```python
from build123d import *

# Parameters (mm, degrees)
F2_R     = 10.5676667099
F3_DEPTH = 124.5231421123
F4_R     = 5.08


# Not quite as in the source:
# - a feature names something its author has since deleted; it is built from what else it names


with BuildPart() as f1:
    # F0 (on Front) → F1 (revolve)
    with BuildSketch(Plane.XZ):
        Polygon((0, 25.3843758255), (0, 0), (124.5221421123, 0), (124.5221421123, 11.6869108751), (108.956836164, 25.3843758255), (94.325453043, 25.3843758255), (94.325453043, 55.5810630322), (84.0523540974, 55.5810630322), (84.0523540974, 25.3843758255), (40.1582047343, 25.3843758255), (40.1582047343, 57.137593627), (28.951190412, 57.137593627), (28.951190412, 25.3843758255), align=None)
    revolve(axis=Axis((62.2610710561, 0, 0), (1, 0, 0)))

    # F2 (on Right) → F3 (cut, through all)
    with BuildSketch(Plane.YZ):
        Circle(F2_R)
    extrude(amount=F3_DEPTH, mode=Mode.SUBTRACT)

    # F4
    f4_edges = [f1.edges().sort_by_distance(p)[0] for p in [
        (108.956836, 0, -25.384376),
        (94.325453, 0, -55.581063),
        (28.95119, 0, -57.137594),
    ]]
    fillet(f4_edges, radius=F4_R)


solid = f1.part
```
Geometry: final body of the model. Coordinates: model frame, mm. A direction names the side the tool comes from. Give positions to 0.01 mm unless a question says otherwise; leave off trailing zeros. Write each loop counter-clockwise with the first axis right and the second up, starting at its lowest first coordinate (ties: lowest second). Pieces come first, ordered by that corner, then holes.
1. Reachability of faces 1 (the cylindrical face through (86.613, -16.695, 53.014)), 2 (the cylindrical face through (14.27, 24.78, -5.5)), 3 (the flat face through (40.158, 25, -12)), 4 (the flat face through (0, 0, 11)) from +Z, -Z, +X, -X, +Y, -Y: full face, straight path, thin tool, end or side. Return the list, or none.
2. Section query A-A, the plane x = 57. Return loops of the section in (y, z).
3. Line query: probe 1 along X at (y, z) = (-25.5, -34); probe 2 along Y at (x, z) = (44, 0). Output: solid intervals per line, ascending.
4. Pin query (flat end, axial travel): P1, Ø8, axis at x = 67.5, z = 21.5, coming from the +Y side; P2, Ø6, axis at x = 46.5, y = -15, coming from the +Z side; P3, Ø4, axis at y = 45, z = 37.5, coming from the -X side. Return the tip coordinate at first contact, or that it passes through.
5. Draft query along Y for faces 5 (the cylindrical face through (100.59, 9.72, 23.45)), 6 (the flat face through (28.951, -12.3, 22.4)), 7 (the cylindrical face through (61.389, -2.291, -10.316)). Return one class per face: released by +Y, released by -Y, zero draft, split by the parting line, or undercut.
Computed:
1. face 1: +X
1. face 2: -X
1. face 3: none
1. face 4: +Z, -Z, -X, +Y, -Y
2. outline: circle Ø50.77 at (0, 0); hole circle Ø21.14 at (0, 0)
3. probe 1: x = 28.95 to 40.16, 84.05 to 94.33
3. probe 2: y = -25.38 to -10.57, 10.57 to 25.38
4. P1: stops at y = 18.39
4. P2: stops at z = 22.37
4. P3: stops at x = 31.71
5. face 5: split by the parting line
5. face 6: zero draft
5. face 7: undercut
